Check sheet for the modelled part. Datum: model origin and axes. Units: mm. Give positions to 0.01 mm unless a question says otherwise; leave off trailing zeros. Order: outer loops, then holes, each group sorted by start corner. A loop starts at its lowest first (then second) coordinate and runs counter-clockwise, first axis right, second up. Notation, with made-up numbers: (58, 49) -> (111, 49) arc R19 cw to (111, 59) -> close; hole circle Ø7 at (30, -18). An arc over 180 degrees is marked (long way). One line per question, with ' | ' between items.
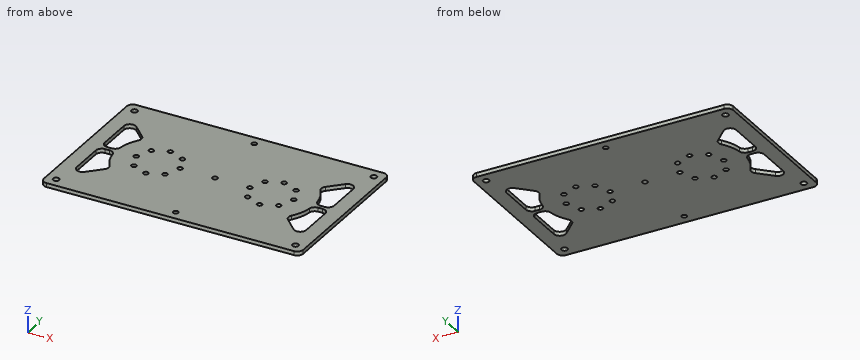
```python
from build123d import *

# Parameters (mm, degrees)
ESBO_O1_W                = 130
ESBO_O1_H                = 80
ESBO_O1_R                = 1.25
ESBO_O1_R_2              = 1.501478649
ESBO_O1_R_3              = 1.5
RESSALTO_EXTRUS_O1_DEPTH = 2
FILETE1_R                = 3
FILETE2_R                = 3


with BuildPart() as part:
    # Esboço1 → Ressalto-extrusão1 (new body)
    with BuildSketch(Plane.XY):
        Rectangle(ESBO_O1_W, ESBO_O1_H)
        with Locations((-39.5, 0)):
            Circle(ESBO_O1_R, mode=Mode.SUBTRACT)
        with Locations((-36.278174593, 7.778174593)):
            Circle(ESBO_O1_R, mode=Mode.SUBTRACT)
        with Locations((-28.5, 11)):
            Circle(ESBO_O1_R, mode=Mode.SUBTRACT)
        with Locations((-20.721825407, 7.778174593)):
            Circle(ESBO_O1_R, mode=Mode.SUBTRACT)
        with Locations((-17.5, 0)):
            Circle(ESBO_O1_R, mode=Mode.SUBTRACT)
        with Locations((-20.721825407, -7.778174593)):
            Circle(ESBO_O1_R, mode=Mode.SUBTRACT)
        with Locations((-28.5, -11)):
            Circle(ESBO_O1_R, mode=Mode.SUBTRACT)
        with Locations((-36.278174593, -7.778174593)):
            Circle(ESBO_O1_R, mode=Mode.SUBTRACT)
        with Locations(Location((39.5, 0, 0), (0, 0, 180))):
            Circle(ESBO_O1_R, mode=Mode.SUBTRACT)
        with Locations(Location((36.278174593, -7.778174593, 0), (0, 0, 180))):
            Circle(ESBO_O1_R, mode=Mode.SUBTRACT)
        with Locations(Location((28.5, -11, 0), (0, 0, 180))):
            Circle(ESBO_O1_R, mode=Mode.SUBTRACT)
        with Locations(Location((20.721825407, -7.778174593, 0), (0, 0, 180))):
            Circle(ESBO_O1_R, mode=Mode.SUBTRACT)
        with Locations(Location((17.5, 0, 0), (0, 0, 180))):
            Circle(ESBO_O1_R, mode=Mode.SUBTRACT)
        with Locations(Location((20.721825407, 7.778174593, 0), (0, 0, 180))):
            Circle(ESBO_O1_R, mode=Mode.SUBTRACT)
        with Locations(Location((28.5, 11, 0), (0, 0, 180))):
            Circle(ESBO_O1_R, mode=Mode.SUBTRACT)
        with Locations(Location((36.278174593, 7.778174593, 0), (0, 0, 180))):
            Circle(ESBO_O1_R, mode=Mode.SUBTRACT)
        with Locations((-60, 35)):
            Circle(ESBO_O1_R_2, mode=Mode.SUBTRACT)
        with Locations((-60, -35)):
            Circle(ESBO_O1_R_2, mode=Mode.SUBTRACT)
        with Locations((60, 35)):
            Circle(ESBO_O1_R_2, mode=Mode.SUBTRACT)
        with Locations((60, -35)):
            Circle(ESBO_O1_R_3, mode=Mode.SUBTRACT)
        Circle(ESBO_O1_R, mode=Mode.SUBTRACT)
        with Locations((0, 35)):
            Circle(ESBO_O1_R, mode=Mode.SUBTRACT)
        with Locations((0, -35)):
            Circle(ESBO_O1_R, mode=Mode.SUBTRACT)
        with BuildLine():
            Line((-57.5, 28.257359313), (-44.008580375, 14.765939688))
            ThreePointArc((-44.008580375, 14.765939688), (-48.076485237, 8.410411341), (-49.5, 1))
            Line((-49.5, 1), (-57.5, 1))
            Line((-57.5, 1), (-57.5, 28.257359313))
        make_face(mode=Mode.SUBTRACT)
        with BuildLine():
            Line((57.5, 28.257359313), (44.008580375, 14.765939688))
            ThreePointArc((44.008580375, 14.765939688), (48.076485237, 8.410411341), (49.5, 1))
            Line((49.5, 1), (57.5, 1))
            Line((57.5, 1), (57.5, 28.257359313))
        make_face(mode=Mode.SUBTRACT)
        with BuildLine():
            Line((57.5, -28.257359313), (44.008580375, -14.765939688))
            ThreePointArc((44.008580375, -14.765939688), (48.076485237, -8.410411341), (49.5, -1))
            Line((49.5, -1), (57.5, -1))
            Line((57.5, -1), (57.5, -28.257359313))
        make_face(mode=Mode.SUBTRACT)
        with BuildLine():
            Line((-57.5, -28.257359313), (-44.008580375, -14.765939688))
            ThreePointArc((-44.008580375, -14.765939688), (-48.076485237, -8.410411341), (-49.5, -1))
            Line((-49.5, -1), (-57.5, -1))
            Line((-57.5, -1), (-57.5, -28.257359313))
        make_face(mode=Mode.SUBTRACT)
    extrude(amount=RESSALTO_EXTRUS_O1_DEPTH)

    # Filete1
    filete1_edges = [part.edges().sort_by_distance(p)[0] for p in [
        (44.008580375, 14.765939688, 1),
        (49.5, 1, 1),
        (57.5, 1, 1),
        (57.5, 28.257359313, 1),
        (49.5, -1, 1),
        (44.008580375, -14.765939688, 1),
        (57.5, -28.257359313, 1),
        (57.5, -1, 1),
        (-44.008580375, -14.765939688, 1),
        (-49.5, -1, 1),
        (-57.5, -1, 1),
        (-57.5, -28.257359313, 1),
        (-49.5, 1, 1),
        (-44.008580375, 14.765939688, 1),
        (-57.5, 28.257359313, 1),
        (-57.5, 1, 1),
    ]]
    fillet(filete1_edges, radius=FILETE1_R)

    # Filete2
    filete2_edges = [part.edges().sort_by_distance(p)[0] for p in [
        (65, -40, 1),
        (-65, -40, 1),
        (-65, 40, 1),
        (65, 40, 1),
    ]]
    fillet(filete2_edges, radius=FILETE2_R)


solid = part.part
```
Q1. Section check A-A (x = 0). Enter the section's corners in (y, z).
Result sheet:
outline: (-40, 0) -> (-36.25, 0) -> (-36.25, 2) -> (-40, 2) -> close; (-33.75, 0) -> (-1.25, 0) -> (-1.25, 2) -> (-33.75, 2) -> close; (1.25, 0) -> (33.75, 0) -> (33.75, 2) -> (1.25, 2) -> close; (36.25, 0) -> (40, 0) -> (40, 2) -> (36.25, 2) -> close
Q2. Section check D-D (z = 0.45). Count the separate pieces of the cut face and the enclosed holes in it, and give its area (3 significant figures).
Result sheet:
separate pieces: 1 | enclosed holes: 27 | area: 9,440 mm2
Q3. Depth check by flat-ended pin: pin 1 Ø2 at (x, y) = (20.72, -7.78) entering from +Z. Enter the tip coordinate at first touch or a pass-through.
Result sheet:
pin 1: passes through
Q4. Section check C-C (y = 15). Enter the section's corners in (x, z), and give its area (3 significant figures).
Result sheet:
outline: (-65, 0) -> (-57.5, 0) -> (-57.5, 2) -> (-65, 2) -> close; (-45.09, 0) -> (45.09, 0) -> (45.09, 2) -> (-45.09, 2) -> close; (57.5, 0) -> (65, 0) -> (65, 2) -> (57.5, 2) -> close | area: 210 mm2
Q5. Thickness scan on line 1 (Y direction, x = 28.5, z = 0.4); line 2 (X direction, y = 23, z = 1.25); line 3 (X direction, y = -21, z = 0.65). Record the ranges inside material, lowest first.
Result sheet:
line 1: y = -40 to -12.25, -9.75 to 9.75, 12.25 to 40 | line 2: x = -65 to -56.75, -52.24 to 52.24, 56.75 to 65 | line 3: x = -65 to -57.5, -50.24 to 50.24, 57.5 to 65
Q6. Section check B-B (x = 60). Enter the section's corners in (y, z).
Result sheet:
outline: (-40, 0) -> (-36.5, 0) -> (-36.5, 2) -> (-40, 2) -> close; (-33.5, 0) -> (33.5, 0) -> (33.5, 2) -> (-33.5, 2) -> close; (36.5, 0) -> (40, 0) -> (40, 2) -> (36.5, 2) -> close
